CAD build for the part. Positions are in the model's coordinates, mm. A direction names the side the tool comes from. Round coordinates to 2 decimals unless told otherwise and drop trailing zeros. Order: outer loops, then holes, each group sorted by start corner. A loop starts at its lowest first (then second) coordinate and runs counter-clockwise, first axis right, second up. Notation, with made-up numbers: M -9.75,-39 L 24.25,-39 A16 ccw 24.25,-28 Z; hole C 39.5,-14 d5. An arc over 180 degrees is marked long. Answer as a JSON object with one key per item and string values.
```python
from build123d import *

# Parameters (mm, degrees)
FILLET_R = 1


with BuildPart() as part:
    # Sketch → Revolution (revolve)
    with BuildSketch(Plane.XY):
        Polygon((21.1, 0), (21.1, 10), (24.57967, 12.115673), (24.92967, 12.115673), (21.45, 10), (21.45, 0), align=None)
    revolve(axis=Axis((0, 0, 0), (0, 1, 0)))

    # Fillet
    fillet_edges = [part.edges().sort_by_distance(p)[0] for p in [
        (-24.57967, 12.115673, 0),
    ]]
    fillet(fillet_edges, radius=FILLET_R)


solid = part.part
```
Item 1: 3-axis set-ups, long thin cutter, end or side, ignore diameter. For faces 4 (the conical face through (-4.618, 10.123, 20.796)), 5 (the cylindrical face through (-15.81, 4.93, -14.497)): which of +Z, -Z, +X, -X, +Y, -Y reach the whole face in a straight line?
Worked answers:
{"face 4": "+Y", "face 5": "-Y"}
Item 2: Drop flat-ended pins along their axis: pin 1 Ø2 at (x, y) = (-11.5, 7.5) entering from +Z; pin 2 Ø6 at (x, y) = (-13, 8) entering from +Z; pin 3 Ø1.5 at (x, y) = (3, 4) entering from -Z. Give the stop position or say it passes through.
Worked answers:
{"pin 1": "stops at z = 18.7", "pin 2": "stops at z = 19.4", "pin 3": "stops at z = -21.33"}
Item 3: Saw through at B-B on z = 0. List the corners of the cut face in (x, y).
Worked answers:
{"outline": "M -24.93,12.12 L -21.45,10 L -21.45,0 L -21.1,0 L -21.1,10 L -24.34,11.97 A1 ccw -24.86,12.12 Z; M 21.1,0 L 21.45,0 L 21.45,10 L 24.93,12.12 L 24.86,12.12 A1 ccw 24.34,11.97 L 21.1,10 Z"}
Item 4: Two-plate mould, pull along X, no slides. Class faces 1 (the conical face through (-4.7, 10.1, 21.1)), 2 (the flat face through (16, 0, 14)), 3 (the cylindrical face through (20.126, 5.07, -6.338)): released by +X, released by -X, zero draft, split by the parting line, or undercut.
Worked answers:
{"face 1": "split by the parting line", "face 2": "zero draft", "face 3": "undercut"}
Item 5: Saw through at C-C on y = 5. List the corners of the cut face in (x, z), and give its area (3 significant figures).
Worked answers:
{"outline": "C 0,0 d42.9; hole C 0,0 d42.2", "area": "46.8 mm2"}
Item 6: Wall check: line 1 along Z through (x, y) = (0, 8.25); line 2 along X through (y, z) = (7, -0.5); line 3 along X through (y, z) = (6.5, 17). Give the ranges that are in metal, low to high. Write a range as [from, to].
Worked answers:
{"line 1": "z = [-21.45, -21.1], [21.1, 21.45]", "line 2": "x = [-21.44, -21.09], [21.09, 21.44]", "line 3": "x = [-13.08, -12.5], [12.5, 13.08]"}
